Read the model definition and answer for the solid it produces. Units are mm, in the model's axes. Face numbers are marked on the shaded views. A direction names the side the tool comes from. Coordinates: 2 decimals unless noted, no trailing zeros. Loops run counter-clockwise (first coordinate to the right, second up) from the corner with the lowest first, then second, coordinate; pieces in that order, holes last. Notation, with made-up numbers: (45.5, -11.5) - (95.5, -11.5) arc R17 ccw to (95.5, 1.5) - close; hole circle Ø1 at (52.25, -32.5). An arc over 180 degrees is marked (long way). Use CSV: the item, a comma, the result in double quotes.
```python
from build123d import *

# Parameters (mm, degrees)
BOSS_EXTRU_1_DEPTH      = 25
ENL_V_MAT_EXTRU_1_DEPTH = 15
ESQUISSE4_R             = 25.355
ENL_V_MAT_EXTRU_2_DEPTH = 255.301687519
ESQUISSE5_R             = 10
BOSS_EXTRU_2_DEPTH      = 30
ENL_V_MAT_EXTRU_3_DEPTH = 264.024268847
CONG_1_R                = 10


with BuildPart() as part:
    # Esquisse1 → Boss.-Extru.1 (new, symmetric)
    with BuildSketch(Plane.XY):
        with BuildLine():
            Line((44.273101825, -200), (44.273101825, -27.730279152))
            ThreePointArc((44.273101825, -27.730279152), (44.686437132, -23.685212253), (45.909358446, -19.807342251))
            ThreePointArc((45.909358446, -19.807342251), (0, 50), (-45.909358446, -19.807342251))
            ThreePointArc((-45.909358446, -19.807342251), (-44.686437132, -23.685212253), (-44.273101825, -27.730279152))
            Line((-44.273101825, -27.730279152), (-44.273101825, -200))
            ThreePointArc((-44.273101825, -200), (0, -244.273101825), (44.273101825, -200))
        make_face()
    extrude(amount=BOSS_EXTRU_1_DEPTH, both=True)

    # Esquisse3 → Enlèv. mat.-Extru.1 (cut, symmetric)
    with BuildSketch(Plane.XY):
        with BuildLine():
            Line((34.273101825, -200), (34.273101825, -38.308494588))
            ThreePointArc((34.273101825, -38.308494588), (36.593682253, -28.957659138), (43.016914187, -21.776760261))
            Line((43.016914187, -21.776760261), (45.909358446, -19.807342251))
            ThreePointArc((45.909358446, -19.807342251), (0, 50), (-45.909358446, -19.807342251))
            Line((-45.909358446, -19.807342251), (-43.016914187, -21.776760261))
            ThreePointArc((-43.016914187, -21.776760261), (-36.593682253, -28.957659138), (-34.273101825, -38.308494588))
            Line((-34.273101825, -38.308494588), (-34.273101825, -200))
            ThreePointArc((-34.273101825, -200), (0, -234.273101825), (34.273101825, -200))
        make_face()
    extrude(amount=ENL_V_MAT_EXTRU_1_DEPTH, both=True, mode=Mode.SUBTRACT)

    # Esquisse4 → Enlèv. mat.-Extru.2 (cut, through all)
    with BuildSketch(Plane.XY.offset(25)):
        with Locations((0, -200)):
            Circle(ESQUISSE4_R)
    extrude(amount=-ENL_V_MAT_EXTRU_2_DEPTH, mode=Mode.SUBTRACT)

    # Esquisse5 → Boss.-Extru.2 (add)
    with BuildSketch(Plane.XY.offset(-15)):
        with Locations(Location((0, 0, 0), (0, 0, 180))):
            Circle(ESQUISSE5_R)
    extrude(amount=BOSS_EXTRU_2_DEPTH)

    # Esquisse6 → Enlèv. mat.-Extru.3 (cut, through all)
    with BuildSketch(Plane.ZY.offset(44.273101825)):
        Polygon((-25, -27.730279152), (-20, -47.730279152), (-20, -248.850889137), (-25, -248.850889137), align=None)
        Polygon((20, -248.850889137), (25, -248.850889137), (25, -27.730279152), (20, -47.730279152), align=None)
    extrude(amount=-ENL_V_MAT_EXTRU_3_DEPTH, mode=Mode.SUBTRACT)

    # Congé1
    cong_1_edges = [part.edges().sort_by_distance(p)[0] for p in [
        (0, -27.730279152, -25),
        (0, -47.730279152, -20),
        (0, -47.730279152, 20),
        (0, -27.730279152, 25),
    ]]
    fillet(cong_1_edges, radius=CONG_1_R)


solid = part.part
```
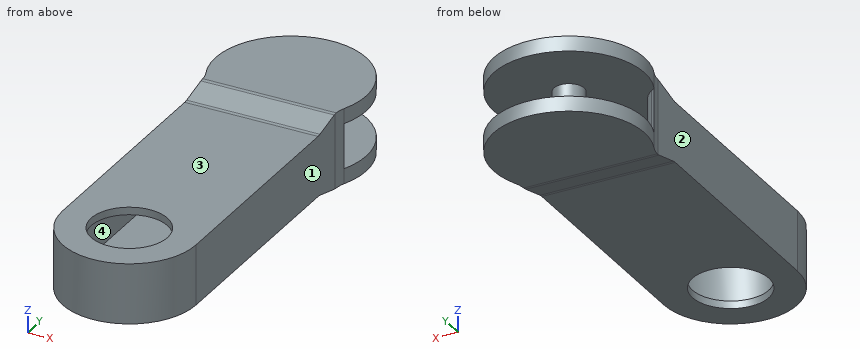
Q1. The part is cut by section C-C on z = 0.5. Determine the outline of the cut face in (x, y).
Reported:
outline,"(-45.91, -19.81) arc R20 cw to (-44.27, -27.73) - (-44.27, -200) arc R44.27 ccw to (44.27, -200) - (44.27, -27.73) arc R20 cw to (45.91, -19.81) - (43.02, -21.78) arc R20 ccw to (34.27, -38.31) - (34.27, -200) arc R34.27 cw to (-34.27, -200) - (-34.27, -38.31) arc R20 ccw to (-43.02, -21.78) - close; circle Ø20 at (0, 0)"
Q2. Find the intervals of material crossed by probe 1 along X at (y, z) = (-119, -2.5); probe 2 along Y at (x, z) = (0, -16) (3 decimals); probe 3 along Z at (x, y) = (-44, 14), in increasing order. Write a range as [from, to].
Reported:
probe 1,"x = [-44.27, -34.27], [34.27, 44.27]"
probe 2,"y = [-244.273, -225.355], [-174.645, 50]"
probe 3,"z = [-25, -15], [15, 25]"
Q3. A tool of negligible diameter and unlimited length cuts with its end or side. For the marked faces 1, 2, 3 and 4, from which of +Z, -Z, +X, -X, +Y, -Y can it reach the whole face along a straight path? Write none if from no direction.
Reported:
face 1,"+Z, -Z, +X, -Y"
face 2,"+Z, -Z, -X, -Y"
face 3,"+Z, +X, -X, -Y"
face 4,"+Y"
Q4. Given P1, Ø5, axis at y = -71, z = 13.5, coming from the +X side; P2, Ø4, axis at y = -87.5, z = -12, coming from the -X side; P3, Ø12, axis at x = -2, z = 19.5, coming from the -Y side, each flat-ended and moving along its own axis, determine where each tip first touches the part or whether it passes through.
Reported:
P1,"stops at x = 44.27"
P2,"stops at x = -44.27"
P3,"stops at y = -244.27"
Q5. The part is cut by section A-A on y = -90.5. Determine the outline of the cut face in (x, z), and give its area (3 significant figures).
Reported:
outline,"(-44.27, -20) - (44.27, -20) - (44.27, 20) - (-44.27, 20) - close; hole (-34.27, -15) - (34.27, -15) - (34.27, 15) - (-34.27, 15) - close"
area,"1,490 mm²"
Q6. The part is cut by section B-B on x = 0. Determine the outline of the cut face in (y, z) (3 decimals).
Reported:
outline,"(-244.273, -20) - (-225.355, -20) - (-225.355, -15) - (-234.273, -15) - (-234.273, 15) - (-225.355, 15) - (-225.355, 20) - (-244.273, 20) - close; (-174.645, -20) - (-48.961, -20) arc R10 cw to (-46.536, -20.299) - (-28.925, -24.701) arc R10 ccw to (-26.499, -25) - (50, -25) - (50, -15) - (10, -15) - (10, 15) - (50, 15) - (50, 25) - (-26.499, 25) arc R10 ccw to (-28.925, 24.701) - (-46.536, 20.299) arc R10 cw to (-48.961, 20) - (-174.645, 20) - (-174.645, 15) - (-10, 15) - (-10, -15) - (-174.645, -15) - close"
Q7. The part is cut by section D-D on x = 38.5. Determine the outline of the cut face in (y, z).
Reported:
outline,"(-221.86, -20) - (-48.96, -20) arc R10 cw to (-46.54, -20.3) - (-28.92, -24.7) arc R10 ccw to (-26.5, -25) - (31.9, -25) - (31.9, -15) - (-26.01, -15) - (-26.01, 15) - (31.9, 15) - (31.9, 25) - (-26.5, 25) arc R10 ccw to (-28.92, 24.7) - (-46.54, 20.3) arc R10 cw to (-48.96, 20) - (-221.86, 20) - close"
